For this review, take the finished solid that the model builds, in its own axes (mm). Coordinates: 2 decimals unless noted, no trailing zeros. Write each loop counter-clockwise with the first axis right and the second up, starting at its lowest first coordinate (ties: lowest second). Pieces come first, ordered by that corner, then holes.
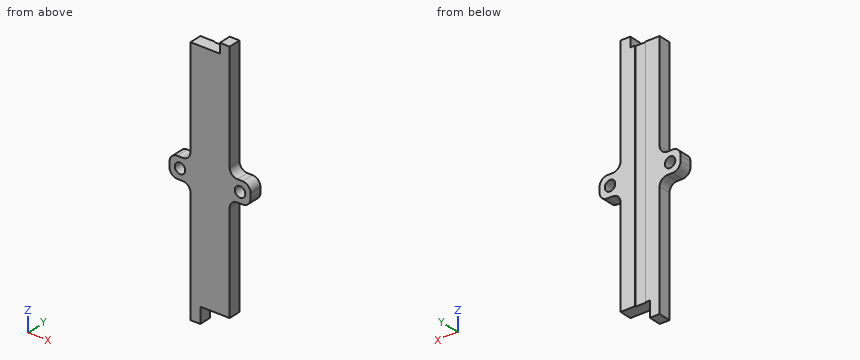
```python
from build123d import *

# Parameters (mm, degrees)
SKETCH1_W               = 12.7
SKETCH1_H               = 4.064
BOSS_EXTRUDE1_DEPTH     = 228.6
SKETCH2_W               = 3.429
SKETCH2_H               = 217.3732
CUT_EXTRUDE1_DEPTH      = 0.254
SKETCH3_W               = 0.508
SKETCH3_H               = 5.08
CUT_EXTRUDE2_DEPTH      = 229.724285103
MIRROR2_COPY_1_SKETCH_W = 0.508
MIRROR2_COPY_1_SKETCH_H = 5.08
MIRROR2_COPY_1_DEPTH    = 229.724285103
SKETCH4_W               = 3.175
SKETCH4_H               = 3.175
CUT_EXTRUDE3_DEPTH      = 229.724285103
CUT_EXTRUDE5_DEPTH      = 229.724285103
SKETCH6_W               = 6.80212
SKETCH6_H               = 6.80212
SKETCH6_R               = 1.70053
BOSS_EXTRUDE2_DEPTH     = 4.064
FILLET1_R               = 2.54


with BuildPart() as part:
    # Sketch1 → Boss-Extrude1 (new body)
    with BuildSketch(Plane.XY):
        Rectangle(SKETCH1_W, SKETCH1_H)
    extrude(amount=BOSS_EXTRUDE1_DEPTH)

    # Sketch2 → Cut-Extrude1 (cut)
    with BuildSketch(Plane(origin=(0, 2.032, 0), x_dir=(1, 0, 0), z_dir=(0, 1, 0))):
        with Locations((0, -114.3)):
            Rectangle(SKETCH2_W, SKETCH2_H)
    extrude(amount=-CUT_EXTRUDE1_DEPTH, mode=Mode.SUBTRACT)

    # Sketch3 → Cut-Extrude2 (cut, through all)
    with BuildSketch(Plane(origin=(0, 2.032, 0), x_dir=(1, 0, 0), z_dir=(0, 1, 0))):
        with Locations((-6.096, -226.06)):
            Rectangle(SKETCH3_W, SKETCH3_H)
    cut_extrude2 = extrude(amount=-CUT_EXTRUDE2_DEPTH, mode=Mode.SUBTRACT)

    # Mirror1: Cut-Extrude2 across plane
    add(cut_extrude2.mirror(Plane(origin=(0, 0, 114.3), x_dir=(1, 0, 0), z_dir=(0, 0, -1))), mode=Mode.SUBTRACT)

    # Mirror2: Cut-Extrude2 across plane
    add(cut_extrude2.mirror(Plane(origin=(0, 0, 0), x_dir=(0, 0, 1), z_dir=(1, 0, 0))), mode=Mode.SUBTRACT)

    # Mirror2 copy 1 sketch → Mirror2 copy 1 (cut, through all)
    with BuildSketch(Plane(origin=(0, 2.032, 228.6), x_dir=(-1, 0, 0), z_dir=(0, 1, 0))):
        with Locations((-6.096, -226.06)):
            Rectangle(MIRROR2_COPY_1_SKETCH_W, MIRROR2_COPY_1_SKETCH_H)
    extrude(amount=-MIRROR2_COPY_1_DEPTH, mode=Mode.SUBTRACT)

    # Sketch4 → Cut-Extrude3 (cut, through all)
    with BuildSketch(Plane(origin=(0, 2.032, 0), x_dir=(1, 0, 0), z_dir=(0, 1, 0))):
        with Locations((-4.2545, -227.0125)):
            Rectangle(SKETCH4_W, SKETCH4_H)
    extrude(amount=-CUT_EXTRUDE3_DEPTH, mode=Mode.SUBTRACT)

    # Sketch5 → Cut-Extrude5 (cut, through all)
    with BuildSketch(Plane(origin=(0, 2.032, 0), x_dir=(1, 0, 0), z_dir=(0, 1, 0))):
        Polygon((-6.35, 0), (6.35, 0), (6.35, -76.2), (-3.175, -76.2), (-3.175, -71.12), (-6.35, -71.12), align=None)
        Polygon((-6.35, -152.4), (3.175, -152.4), (3.175, -155.575), (6.35, -155.575), (6.35, -228.6), (-6.35, -228.6), align=None)
    extrude(amount=-CUT_EXTRUDE5_DEPTH, mode=Mode.SUBTRACT)

    # Sketch6 → Boss-Extrude2 (add, through all)
    # profile 1 of 2: a face of its own
    with BuildSketch(Plane(origin=(0, 2.032, 0), x_dir=(1, 0, 0), z_dir=(0, 1, 0))):
        with Locations((-9.75106, -114.3)):
            Rectangle(SKETCH6_W, SKETCH6_H)
        with Locations(Location((-9.75106, -114.3, 0), (0, 0, 270))):
            Circle(SKETCH6_R, mode=Mode.SUBTRACT)
    # profile 2 of 2: a face of its own
    with BuildSketch(Plane(origin=(0, 2.032, 0), x_dir=(1, 0, 0), z_dir=(0, 1, 0))):
        with Locations((9.75106, -114.3)):
            Rectangle(SKETCH6_W, SKETCH6_H)
        with Locations(Location((9.75106, -114.3, 0), (0, 0, 270))):
            Circle(SKETCH6_R, mode=Mode.SUBTRACT)
    extrude(amount=-BOSS_EXTRUDE2_DEPTH)

    # Fillet1
    fillet1_edges = [part.edges().sort_by_distance(p)[0] for p in [
        (6.35, 0, 110.89894),
        (13.15212, 0, 110.89894),
        (13.15212, 0, 117.70106),
        (6.35, 0, 117.70106),
        (-6.35, 0, 117.70106),
        (-13.15212, 0, 117.70106),
        (-13.15212, 0, 110.89894),
        (-6.35, 0, 110.89894),
    ]]
    fillet(fillet1_edges, radius=FILLET1_R)


solid = part.part
```
1) Consider section A-A (z = 114.3). Give the boundary of the cut face in (x, y), then the cut area to 3 significant figures.
2) Clearance check with flat-ended pins moving along their axes: P1, Ø1.5, axis at x = 9.5, y = 1.5, coming from the +Z side; P2, Ø1, axis at y = 1, z = 106.5, coming from the +X side; P3, Ø1.2, axis at y = -0.5, z = 143, coming from the -X side; P4, Ø3, axis at x = 9.75, z = 114.3, coming from the +Y side. State where each tip first meets the part, or that it passes through.
3) For L1, parallel to X at y = 0.8, z = 114.3; L2, parallel to Z at x = 10, y = 1.3; L3, parallel to Z at x = -2.5, y = 1.75, list the stretches that pass through material, from the lowest coordinate up.
4) Consider section B-B (y = 0.3). Give the boundary of the cut face in (x, z) (3 decimals), then the cut area to 3 significant figures.
5) Consider section D-D (x = -0.5). Give the boundary of the cut face in (y, z), then the cut area to 3 significant figures.
6) Consider section C-C (z = 91.5). Give the boundary of the cut face in (x, y), then the cut area to 3 significant figures.
Results:
1. outline: (-13.15, -2.03) - (-11.45, -2.03) - (-11.45, 2.03) - (-13.15, 2.03) - close; (-8.05, -2.03) - (8.05, -2.03) - (8.05, 2.03) - (1.71, 2.03) - (1.71, 1.78) - (-1.71, 1.78) - (-1.71, 2.03) - (-8.05, 2.03) - close; (11.45, -2.03) - (13.15, -2.03) - (13.15, 2.03) - (11.45, 2.03) - close
1. area: 78.4 mm2
2. P1: stops at z = 117.7
2. P2: stops at x = 6.35
2. P3: stops at x = -6.35
2. P4: passes through
3. L1: x = -13.15 to -11.45, -8.05 to 8.05, 11.45 to 13.15
3. L2: z = 110.9 to 112.62, 115.98 to 117.7
3. L3: z = 76.2 to 152.4
4. outline: (-13.152, 113.439) arc R2.54 ccw to (-10.612, 110.899) - (-8.89, 110.899) arc R2.54 cw to (-6.35, 108.359) - (-6.35, 71.12) - (-3.175, 71.12) - (-3.175, 76.2) - (6.35, 76.2) - (6.35, 108.359) arc R2.54 cw to (8.89, 110.899) - (10.612, 110.899) arc R2.54 ccw to (13.152, 113.439) - (13.152, 115.161) arc R2.54 ccw to (10.612, 117.701) - (8.89, 117.701) arc R2.54 cw to (6.35, 120.241) - (6.35, 155.575) - (3.175, 155.575) - (3.175, 152.4) - (-6.35, 152.4) - (-6.35, 120.241) arc R2.54 cw to (-8.89, 117.701) - (-10.612, 117.701) arc R2.54 ccw to (-13.152, 115.161) - close; hole circle Ø3.401 at (-9.751, 114.3); hole circle Ø3.401 at (9.751, 114.3)
4. area: 1,070 mm2
5. outline: (-2.03, 76.2) - (1.78, 76.2) - (1.78, 152.4) - (-2.03, 152.4) - close
5. area: 290 mm2
6. outline: (-6.35, -2.03) - (6.35, -2.03) - (6.35, 2.03) - (1.71, 2.03) - (1.71, 1.78) - (-1.71, 1.78) - (-1.71, 2.03) - (-6.35, 2.03) - close
6. area: 50.7 mm2
